```python
from build123d import *

# Parameters (mm, degrees)
SKETCH1_R             = 38
BOSS_EXTRUDE1_DEPTH   = 600
BOSS_EXTRUDE1_2_DEPTH = 600
BOSS_EXTRUDE1_3_DEPTH = 600
BOSS_EXTRUDE1_4_DEPTH = 600
BOSS_EXTRUDE1_5_DEPTH = 600
SKETCH2_R             = 110
BOSS_EXTRUDE2_DEPTH   = 140


with BuildPart() as part:
    # Sketch1 → Boss-Extrude1 (new body)
    with BuildSketch(Plane(origin=(0, 0, 0), x_dir=(1, 0, 0), z_dir=(0, 1, 0))):
        with Locations(Location((65.370232552, 21.240076103, 0), (0, 0, 270))):
            Circle(SKETCH1_R)
    extrude(amount=BOSS_EXTRUDE1_DEPTH)



with BuildPart() as body_2:
    # Sketch1 → Boss-Extrude1 2 (new body)
    with BuildSketch(Plane(origin=(0, 0, 0), x_dir=(1, 0, 0), z_dir=(0, 1, 0))):
        with Locations(Location((40.401025569, -55.607241162, 0), (0, 0, 270))):
            Circle(SKETCH1_R)
    extrude(amount=BOSS_EXTRUDE1_2_DEPTH)


with BuildPart() as body_3:
    # Sketch1 → Boss-Extrude1 3 (new body)
    with BuildSketch(Plane(origin=(0, 0, 0), x_dir=(1, 0, 0), z_dir=(0, 1, 0))):
        with Locations(Location((-40.401025569, -55.607241162, 0), (0, 0, 270))):
            Circle(SKETCH1_R)
    extrude(amount=BOSS_EXTRUDE1_3_DEPTH)


with BuildPart() as body_4:
    # Sketch1 → Boss-Extrude1 4 (new body)
    with BuildSketch(Plane(origin=(0, 0, 0), x_dir=(1, 0, 0), z_dir=(0, 1, 0))):
        with Locations(Location((-65.370232552, 21.240076103, 0), (0, 0, 270))):
            Circle(SKETCH1_R)
    extrude(amount=BOSS_EXTRUDE1_4_DEPTH)


with BuildPart() as body_5:
    # Sketch1 → Boss-Extrude1 5 (new body)
    with BuildSketch(Plane(origin=(0, 0, 0), x_dir=(1, 0, 0), z_dir=(0, 1, 0))):
        with Locations(Location((0, 68.734330118, 0), (0, 0, 270))):
            Circle(SKETCH1_R)
    extrude(amount=BOSS_EXTRUDE1_5_DEPTH)


with BuildPart() as part_1:
    add(part.part)

    add(body_2.part)  # Boss-Extrude2 merges body 2

    add(body_3.part)  # Boss-Extrude2 merges body 3

    add(body_4.part)  # Boss-Extrude2 merges body 4

    add(body_5.part)  # Boss-Extrude2 merges body 5
    # Sketch2 → Boss-Extrude2 (add)
    with BuildSketch(Plane.XZ):
        with Locations(Location((0, 0, 0), (0, 0, 270))):
            Circle(SKETCH2_R)
    extrude(amount=BOSS_EXTRUDE2_DEPTH)


solid = part_1.part
```
CAD build for the part. Positions are in the model's coordinates, mm. A direction names the side the tool comes from. Give positions to 0.01 mm unless a question says otherwise; leave off trailing zeros. Order: outer loops, then holes, each group sorted by start corner. A loop starts at its lowest first (then second) coordinate and runs counter-clockwise, first axis right, second up.
(1) Saw through at D-D, the plane y = -73. Give the cut face in (x, z).
(2) Saw through at A-A, the plane y = 12.5. Give the cut face in (x, z), then the cut area to 3 significant figures.
(3) Saw through at C-C, the plane x = 96.5. Give the cut face in (y, z), then the cut area to 3 significant figures.
(4) Tool access for faces 4 (the flat face through (2, -140, 2)), 5 (the cylindrical face through (51.82, 295.8, 91.85)): list every direction of +Z, -Z, +X, -X, +Y, -Y with a clear straight run to the whole face (end or side of a thin tool).
(5) Mould opens along Z. For faces 1 (the flat face through (-8, 0, 1)), 2 (the cylindrical face through (-97.59, -69.02, -50.76)), 3 (the flat face through (66, 600, -22)) say: released by +Z, released by -Z, zero draft, split by the parting line, or undercut.
(6) Saw through at B-B, the plane z = 0. Give the cut face in (x, y).
(7) Drill centre lines: L1, parallel to X at y = 363.5, z = -39; L2, parallel to X at y = 145, z = 56.5; L3, parallel to Z at x = -8, y = 519. Where is each one in solid material? Low to high.
(8) Flat gauge pins, fed straight in: pin 1 (5 mm diameter, centred on y = 15.5, z = -50.5, fed in from -X); pin 2 (10 mm diameter, centred on y = 218, z = -51, fed in from +X); pin 3 (3 mm diameter, centred on x = -28, y = 388.5, fed in from +Z). Where does each tip first touch, or does it go through?
Results found:
1. outline: circle Ø220 at (0, 0)
2. outline: circle Ø76 at (-65.37, -21.24); circle Ø76 at (-40.4, 55.61); circle Ø76 at (0, -68.73); circle Ø76 at (40.4, 55.61); circle Ø76 at (65.37, -21.24)
2. area: 22,700 mm2
3. outline: (-140, -52.8) - (0, -52.8) - (0, -43.03) - (600, -43.03) - (600, 0.55) - (0, 0.55) - (0, 52.8) - (-140, 52.8) - close
3. area: 40,900 mm2
4. face 4: +Z, -Z, +X, -X, -Y
4. face 5: +Y
5. face 1: undercut
5. face 2: split by the parting line
5. face 3: zero draft
6. outline: (-110, -140) - (110, -140) - (110, 0) - (96.88, 0) - (96.88, 600) - (33.86, 600) - (33.86, 0) - (-33.86, 0) - (-33.86, 600) - (-96.88, 600) - (-96.88, 0) - (-110, 0) - close
7. L1: x = -98.96 to -31.78, -23.66 to 23.66, 31.78 to 98.96
7. L2: x = -78.39 to -2.41, 2.41 to 78.39
7. L3: z = -105.88 to -31.59, 35.75 to 75.46
8. pin 1: stops at x = -92.35
8. pin 2: stops at x = 94.2
8. pin 3: stops at z = 92.01
